The model under review builds one solid part; all positions refer to its coordinate system, in mm. A direction names the side the tool comes from. Round coordinates to 2 decimals unless told otherwise and drop trailing zeros. Write each loop counter-clockwise with the first axis right and the second up, starting at its lowest first coordinate (ties: lowest second). Pieces come first, ordered by that corner, then holes. Notation, with made-up numbers: M 35.25,54.25 L 94.25,54.25 A32 ccw 94.25,91.25 Z; hole C -15.5,23 d11. An arc over 180 degrees is marked long. Write item = value, one per line. Start each with the question number.
Item 1: Take a section at B-B, the plane y = -0.75. Give the boundary of the cut face in (x, z), plus the area to 3 significant figures.
Item 2: The part is to be moulded in two halves that separate along Y. For faces 6 (the flat face through (19.5, -3, 0.5)), 7 (the flat face through (5.5, -6, 1)), 8 (the flat face through (2, -4, 1)), say which applies: +Y half, -Y half, draft (parallel to the pull), parting line (faces both ways), or undercut.
Item 3: Take a section at C-C, the plane x = 4.25. Give the boundary of the cut face in (y, z).
Item 4: Tool access review of faces 1 (the flat face through (14, -10, 1)), 2 (the flat face through (23, -3, 1)), 3 (the flat face through (20.5, -6, 1)), 4 (the flat face through (1.5, -6, 1)), 5 (the flat face through (4, -5, 2)): name each direction out of +Z, -Z, +X, -X, +Y, -Y from which nothing blocks a thin tool from reaching the whole face with its end or side.
Item 5: To check wall thickness, follow line 1 along X through (y, z) = (-3.75, 0.25); line 2 along X through (y, z) = (-7.25, 2.2); line 3 along X through (y, z) = (-3.5, 2.85). State the ranges of each line that lie inside material, in increasing order.
Item 6: Take a section at D-D, the plane x = 15.75. Give the boundary of the cut face in (y, z), plus the area to 3 significant figures.
Item 7: For pin 1 Ø1 at (x, z) = (22, 1.5) entering from +Y; pin 2 Ø1 at (x, z) = (13, 0.5) entering from +Y; pin 3 Ø0.6 at (x, y) = (4.5, -4.5) entering from +Z, all flat-tipped, find the tip position at first contact; note any pin that passes through.
Autodesk Fusion 360 part; units mm, degrees
sketch "Base" plane through (0, 0, 0) normal (0, 0, 1) x (1, 0, 0)
  line L0 (0, 0) -> (0, -9.0622)
  line L1 (24, -10) -> (24, -3)
  line L2 (22.5, -4) -> (22.5, -8)
  line L3 (20.5, -5) -> (3.5, -5)
  line L4 (1.5, -8) -> (1.5, -4)
  line L5 (1.5, 0) -> (0, 0)
  line L6 (3.5, -5) -> (3.5, -8)
  line L7 (3.5, -8) -> (1.5, -8)
  line L8 (22.5, -8) -> (20.5, -8)
  line L9 (20.5, -5) -> (20.5, -8)
  line L10 (24, -3) -> (21, -3)
  line L11 (21, -3) -> (21, -4)
  line L12 (21, -4) -> (22.5, -4)
  line L13 (1.5, 0) -> (2.5, -3)
  line L14 (2.5, -3) -> (2.5, -4)
  line L15 (2.5, -4) -> (1.5, -4)
  line L16 (21, -4) -> (2.5, -4) construction
  line L17 (3.5, -10) -> (0, -9.0622)
  line L18 (3.5, -8) -> (3.5, -10) construction
  line L19 (3.5, -10) -> (24, -10)
  dimension "d4" = 21
  dimension "d5" = 3.5
  dimension "d7" = 2
  dimension "d8" = 2
  dimension "d10" = 1
  dimension "d11" = 3
  dimension "d15" = 1
  dimension "d16" = 4
  dimension "d17" = 4
  dimension "d18" = 2.5
  dimension "d19" = 1.5
  dimension "d20" = 3
  dimension "d48" = 6
  dimension "d49" = 165
  dimension "d50" = 1.5
extrude "Extrude1" add sketch "Base" along normal blind 3
sketch "Cutout" plane through (0, -5, 0) normal (0, 1, 0) x (-1, 0, 0)
  line L0 (-20.5, 0) -> (-3.5, 0)
  line L1 (-3.5, 0) -> (-3.5, 3)
  line L2 (-3.5, 3) -> (-20.5, 3)
  line L3 (-20.5, 3) -> (-20.5, 0)
  line L4 (-5.5, 0) -> (-18.5, 0)
  line L5 (-18.5, 0) -> (-18.5, 3)
  line L6 (-18.5, 3) -> (-5.5, 3)
  line L7 (-5.5, 3) -> (-5.5, 0)
  dimension "d31" = 13
extrude "Extrude2" cut sketch "Cutout" against normal blind 3 contours L0 L2 L4 L5 L6 L7
sketch "Stand" plane through (0, -5, 0) normal (0, 1, 0) x (-1, 0, 0)
  line L0 (-5.5, 3) -> (-5.5, 0)
  line L1 (-5.5, 0) -> (-3.5, 0)
  line L2 (-3.5, 0) -> (-3.5, 3)
  line L3 (-3.5, 3) -> (-5.5, 3)
  line L4 (-3.5, 0) -> (-5.5, 0)
  line L5 (-5.5, 0) -> (-5.5, 1)
  line L6 (-5.5, 1) -> (-3.5, 1)
  line L7 (-3.5, 1) -> (-3.5, 0)
  dimension "d32" = 1
sketch "Stand (1)" plane through (0, -5, 0) normal (0, 1, 0) x (-1, 0, 0)
  line L0 (-18.5, 0) -> (-18.5, 3)
  line L1 (-18.5, 3) -> (-20.5, 3)
  line L2 (-20.5, 3) -> (-20.5, 0)
  line L3 (-20.5, 0) -> (-18.5, 0)
  line L4 (-18.5, 0) -> (-20.5, 0)
  line L5 (-20.5, 0) -> (-20.5, 1)
  line L6 (-20.5, 1) -> (-18.5, 1)
  line L7 (-18.5, 1) -> (-18.5, 0)
  dimension "d33" = 1
extrude "Extrude3" add sketch "Stand" sketch "Stand (1)" along normal blind 2 contours L0 L1 L2 L4 L5 L6 L7 of sketch 2 contours L0 L2 L3 L4 L5 L6 L7
fillet "Fillet1" radius 0.5 9 edges at (5.5, -3, 0.5) (5.5, -5, 2) (18.5, -5, 2) (18.5, -3, 0.5) (20.5, -3, 0.5) (3.5, -3, 0.5) (0, 0, 1.5) (24, -3, 1.5) (21, -3, 1.5)
fillet "Fillet1" radius 0.75 3 edges at (1.5, -8, 1.5) (20.5, -8, 1.5) (3.5, -8, 1.5)
equation "CLIP_PCB_SIZE = 21 mm"
equation "d4 = CLIP_PCB_SIZE"
equation "d31 = CLIP_PCB_SIZE - 8 mm"
Response values:
q1.outline = M 0,0 L 1.75,0 L 1.75,3 L 0,3 Z
q1.area = 5.25 mm2
q2.face_6 = +Y half
q2.face_7 = draft
q2.face_8 = undercut
q3.outline = M -10,0 L -3,0 L -3,1 L -5,1 L -5,3 L -10,3 Z
q4.face_1 = +Z, -Z, +X, -X, -Y
q4.face_2 = +Z, -Z, +X, +Y
q4.face_3 = +Z, -Z, +Y
q4.face_4 = +Z, -Z
q4.face_5 = +Z, +Y
q5.line_1 = 0 to 2.5, 3.5 to 5.5, 18.5 to 20.5, 21 to 24
q5.line_2 = 0 to 1.5, 3.5 to 5.5, 18.5 to 20.5, 22.5 to 24
q5.line_3 = 0 to 2.5, 21 to 24
q6.outline = M -10,0 L -8,0 L -8,3 L -10,3 Z
q6.area = 6.00 mm2
q7.pin_1 = -3
q7.pin_2 = -8
q7.pin_3 = 1
